The figure shows three views and two pictorial views of one solid part (mm, origin at its lowest corner). Answer the questions. Coordinates: 2 decimals unless noted, no trailing zeros. Loops run counter-clockwise (first coordinate to the right, second up) from the corner with the lowest first, then second, coordinate; pieces in that order, holes last.
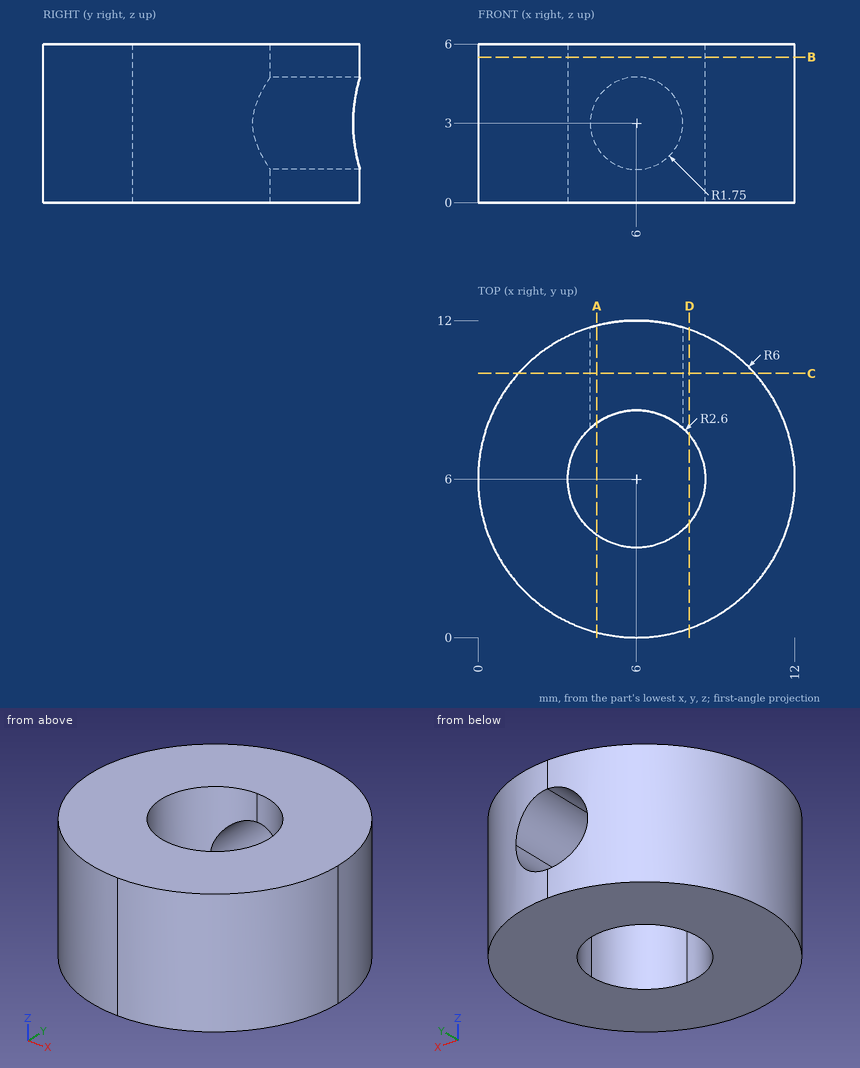
1. A cutting plane is placed at D-D, the plane x = 8. Give the vertices of the cut face in (y, z).
2. A cutting plane is placed at C-C, the plane y = 10. Give the vertices of the cut face in (x, z), then the cut area to 3 significant figures.
3. Straight lines are drawn through the part: probe 1 along X at (y, z) = (8.5, 2.5); probe 2 along X at (y, z) = (7.25, 1.75); probe 3 along Y at (x, z) = (5.25, 4.75). For each, find the intervals that lie inside material, in ascending order.
4. A cutting plane is placed at B-B, the plane z = 5.5. Give the vertices of the cut face in (x, y), then the cut area to 3 significant figures.
5. A cutting plane is placed at A-A, the plane x = 4.5. Give the vertices of the cut face in (y, z), then the cut area to 3 significant figures.
6. Each of these flat-tipped pins is pushed along its axis until it touches: P1, Ø1, axis at y = 1.5, z = 1.5, coming from the -X side; P2, Ø2, axis at x = 6.5, z = 2.5, coming from the +Y side. Where does it stop, or does it pass through?
Answers below:
1. outline: (0.34, 0) - (4.34, 0) - (4.34, 6) - (0.34, 6) - close; (7.66, 0) - (11.66, 0) - (11.66, 6) - (7.66, 6) - close
2. outline: (1.53, 0) - (10.47, 0) - (10.47, 6) - (1.53, 6) - close; hole circle Ø3.5 at (6, 3)
2. area: 44.0 mm2
3. probe 1: x = 0.55 to 4.32, 7.68 to 11.45
3. probe 2: x = 0.13 to 3.72, 8.28 to 11.87
3. probe 3: y = 0.05 to 3.51, 8.49 to 11.95
4. outline: circle Ø12 at (6, 6); hole circle Ø5.2 at (6, 6)
4. area: 91.9 mm2
5. outline: (0.19, 0) - (3.88, 0) - (3.88, 6) - (0.19, 6) - close; (8.12, 0) - (11.81, 0) - (11.81, 2.1) - (8.12, 2.1) - close; (8.12, 3.9) - (11.81, 3.9) - (11.81, 6) - (8.12, 6) - close
5. area: 37.6 mm2
6. P1: stops at x = 1.53
6. P2: stops at y = 3.88
